Check sheet for the modelled part. Datum: model origin and axes. Units: mm. Face numbers are marked on the shaded views. A direction names the side the tool comes from. Round coordinates to 2 decimals unless told otherwise and drop trailing zeros. Write each loop counter-clockwise with the first axis right and the second up, starting at its lowest first coordinate (ties: lowest second). Pieces come first, ordered by that corner, then holes. Notation, with made-up numbers: (74.25, -9.5) - (115.25, -9.5) arc R5 ccw to (115.25, -1.5) - close; hole circle Ø3 at (32.5, 43). An arc over 180 degrees is marked (long way). Answer as a JSON object with one key per item and string values. Group by question number.
Item 1: Sectioned sample at B-B on y = 50. Record the boundary of the cut face in (x, z).
Item 2: Sectioned sample at D-D on z = -90.5. Record the boundary of the cut face in (x, y), plus the area to 3 significant figures.
Item 3: Thickness scan on line 1 (Y direction, x = -46, z = 75); line 2 (X direction, y = 17, z = 65.5); line 3 (Z direction, x = 28.5, y = 33.5). Record the ranges inside material, lowest first.
Item 4: Sectioned sample at A-A on z = 75. Record the boundary of the cut face in (x, y).
Item 5: Sectioned sample at C-C on x = -37.5. Record the boundary of the cut face in (y, z), plus the area to 3 significant figures.
Item 6: Release check for a two-part mould opening along X. For the marked faces 6, 7 and 8 record: pulls with the +X half, pulls with the -X half, needs draft (parallel to the pull), parting line crosses it, or undercut.
Item 7: Gauge pin test, flat ends, axial feed: P1, Ø14, axis at y = 47, z = -77, coming from the -X side; P2, Ø5, axis at x = 7.5, z = -54, coming from the -Y side (3 decimals); P3, Ø10, axis at x = -44, y = 38.5, coming from the +Z side; P4, Ø3, axis at x = -23.5, y = 45.5, coming from the -Z side. Record the tip position at first contact, or that the pin passes through.
Item 8: Set-up check for the marked faces 1, 2, 3, 4 and 5: record each of +Z, -Z, +X, -X, +Y, -Y from which the full face is reachable in a straight line by a thin tool's end or side.
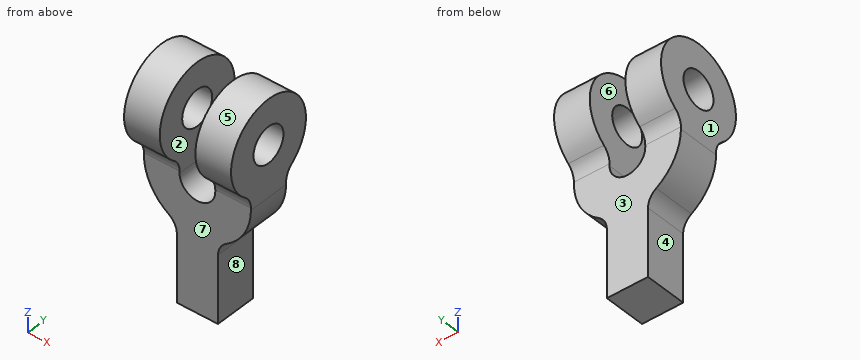
```python
from build123d import *

# Parameters (mm, degrees)
SKETCH2_W           = 120
SKETCH2_H           = 250
BOSS_EXTRUDE1_DEPTH = 100
SKETCH4_R           = 20
CUT_EXTRUDE1_DEPTH  = 100
SKETCH5_R           = 20
CUT_EXTRUDE5_DEPTH  = 201.062490237


with BuildPart() as part:
    # Sketch2 → Boss-Extrude1 (new body)
    with BuildSketch(Plane(origin=(0, 0, 0), x_dir=(1, 0, 0), z_dir=(0, 1, 0))):
        Rectangle(SKETCH2_W, SKETCH2_H)
    extrude(amount=BOSS_EXTRUDE1_DEPTH)

    # Sketch4 → Cut-Extrude1 (cut)
    with BuildSketch(Plane(origin=(0, 100, 0), x_dir=(1, 0, 0), z_dir=(0, 1, 0))):
        with BuildLine():
            Line((-60, 125), (-60, -17.644609552))
            ThreePointArc((-60, -17.644609552), (-52.622366518, 11.180492718), (-32.303782241, 32.916893747))
            ThreePointArc((-32.303782241, 32.916893747), (-25.530920786, 40.16236081), (-23.071709655, 49.770728302))
            Line((-23.071709655, 49.770728302), (-23.071709655, 125))
            Line((-23.071709655, 125), (-60, 125))
        make_face()
        with BuildLine():
            ThreePointArc((32.303782241, 32.916893747), (52.62236667, 11.18049244), (60, -17.644610185))
            Line((60, -17.644610185), (60, 125))
            Line((60, 125), (23.071709655, 125))
            Line((23.071709655, 125), (23.071709655, 49.770728302))
            ThreePointArc((23.071709655, 49.770728302), (25.530920786, 40.16236081), (32.303782241, 32.916893747))
        make_face()
        with Locations((0, -17.644609919)):
            Circle(SKETCH4_R)
        with BuildLine():
            Line((-20, -17.644609919), (-20, -74.213152414))
            ThreePointArc((-20, -74.213152414), (0, -77.644609919), (20, -74.213152414))
            Line((20, -74.213152414), (20, -17.644609919))
            ThreePointArc((20, -17.644609919), (0, -37.644609919), (-20, -17.644609919))
        make_face()
        with BuildLine():
            Line((-20, -74.213152414), (-20, -125))
            Line((-20, -125), (20, -125))
            Line((20, -125), (20, -74.213152414))
            ThreePointArc((20, -74.213152414), (0, -77.644609919), (-20, -74.213152414))
        make_face()
    extrude(amount=-CUT_EXTRUDE1_DEPTH, mode=Mode.SUBTRACT)

    # Sketch5 → Cut-Extrude5 (cut, through all)
    # profile 1 of 2: a face of its own
    with BuildSketch(Plane(origin=(60, 0, 0), x_dir=(0, 0, -1), z_dir=(1, 0, 0))):
        Polygon((125, 100), (49.770728302, 100), (32.916893747, 100), (-17.644609919, 100), (-125, 100), (-125, 0), (-17.644609919, 0), (32.916893747, 0), (49.770728302, 0), (125, 0), align=None)
        with BuildLine():
            Line((125, 73.474979738), (125, 26.525020262))
            Line((125, 26.525020262), (-20.137206262, 26.525020262))
            ThreePointArc((-20.137206262, 26.525020262), (-28.84270867, 24.530970051), (-35.812290187, 18.946443044))
            ThreePointArc((-35.812290187, 18.946443044), (-125, 50), (-35.812290187, 81.053556956))
            ThreePointArc((-35.812290187, 81.053556956), (-28.84270867, 75.469029949), (-20.137206262, 73.474979738))
            Line((-20.137206262, 73.474979738), (125, 73.474979738))
        make_face(mode=Mode.SUBTRACT)
    # profile 2 of 2: a face of its own
    with BuildSketch(Plane(origin=(60, 0, 0), x_dir=(0, 0, -1), z_dir=(1, 0, 0))):
        with Locations((-75, 50)):
            Circle(SKETCH5_R)
    extrude(amount=-CUT_EXTRUDE5_DEPTH, mode=Mode.SUBTRACT)


with BuildPart() as cut_extrude5_kept_piece:
    # of the separate pieces the step leaves, the one the design keeps (cut_extrude5_pieces_kept)
    add(part.part.solids().sort_by_distance((23.071709655, 73.474979738, -125))[0])


solid = cut_extrude5_kept_piece.part
```
Completed:
{
 "1": {"outline": "(-60, 17.64) arc R60 ccw to (-32.3, -32.92) arc R20 cw to (-23.07, -49.77) - (-23.07, -125) - (23.07, -125) - (23.07, -49.77) arc R20 cw to (32.3, -32.92) arc R60 ccw to (60, 17.64) - (60, 55) - (20, 55) - (20, 17.64) arc R20 cw to (-20, 17.64) - (-20, 55) - (-60, 55) - close; (-60, 95) - (-20, 95) - (-20, 125) - (-60, 125) - close; (20, 95) - (60, 95) - (60, 125) - (20, 125) - close"},
 "2": {"outline": "(-23.07, 26.53) - (23.07, 26.53) - (23.07, 73.47) - (-23.07, 73.47) - close", "area": "2,170 mm²"},
 "3": {"line 1": "0 to 30, 70 to 100", "line 2": "-60 to -20, 20 to 60", "line 3": "-36.07 to 63.7, 86.3 to 122.2"},
 "4": {"outline": "(-60, 0) - (-20, 0) - (-20, 30) - (-60, 30) - close; (-60, 70) - (-20, 70) - (-20, 100) - (-60, 100) - close; (20, 0) - (60, 0) - (60, 30) - (20, 30) - close; (20, 70) - (60, 70) - (60, 100) - (20, 100) - close"},
 "5": {"outline": "(18.95, 35.81) arc R20 cw to (26.53, 20.14) - (26.53, -29.19) - (73.47, -29.19) - (73.47, 20.14) arc R20 cw to (81.05, 35.81) arc R50 ccw (long way) to start; hole circle Ø40 at (50, 75)", "area": "9,260 mm²"},
 "6": {"face 6": "undercut", "face 7": "needs draft", "face 8": "pulls with the +X half"},
 "7": {"P1": "x = -23.07", "P2": "y = 26.525", "P3": "z = 124.58", "P4": "z = -125"},
 "8": {"face 1": "+Z, -Z, -X, +Y, -Y", "face 2": "+Z, +Y, -Y", "face 3": "-Z, +X, -X, +Y", "face 4": "-Z, -X, +Y, -Y", "face 5": "+X, -X"}
}
